Verification items for this drawing (mm, ordinates from the low corner). A direction names the side the tool comes from. Round coordinates to 2 decimals unless told otherwise and drop trailing zeros. Loops run counter-clockwise (first coordinate to the right, second up) from the corner with the lowest first, then second, coordinate; pieces in that order, holes last. Notation, with made-up numbers: (-10.5, 36.5) -> (23.5, 36.5) arc R14 cw to (23.5, 42.5) -> close; hole circle Ø4 at (35, -28.75). An arc over 180 degrees is marked (long way). One line per question, with ' | ' between items.
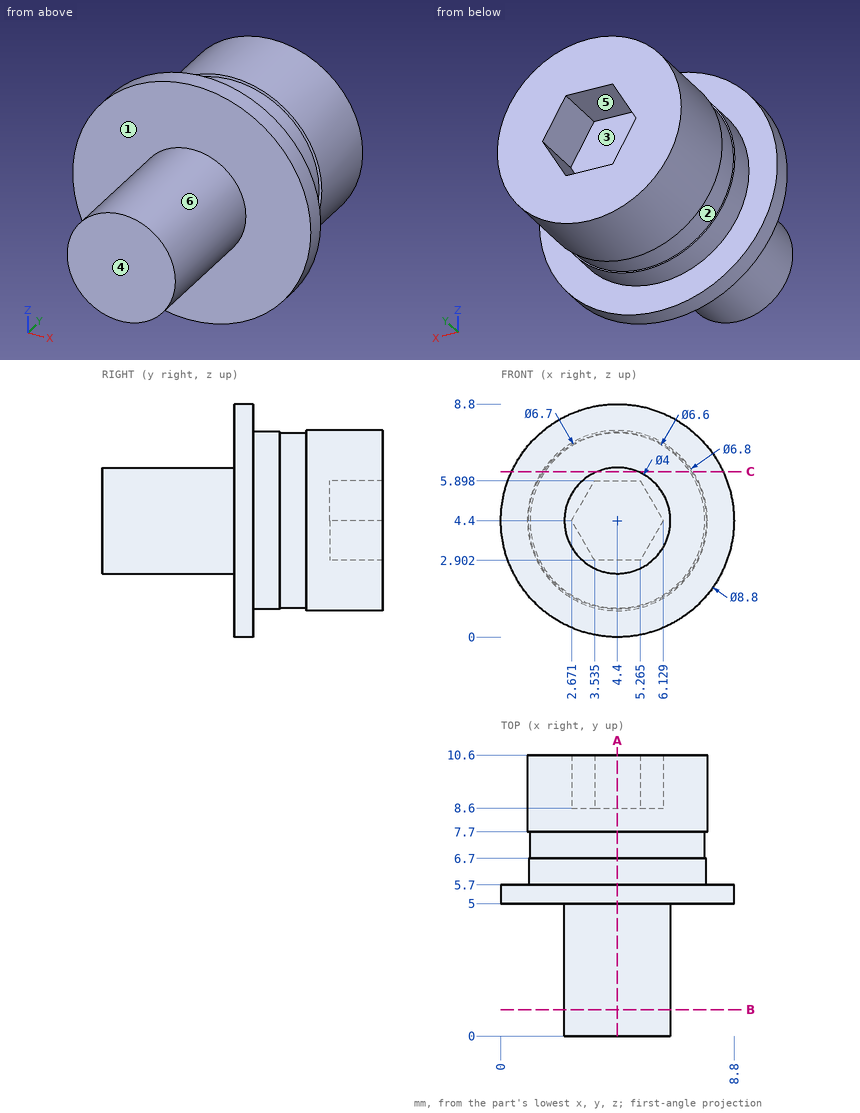
(1) Sectioned sample at A-A, the plane x = 4.4. Record the cut outline in (y, z).
Answer:
outline: (0, 2.4) -> (5, 2.4) -> (5, 0) -> (5.7, 0) -> (5.7, 1.05) -> (6.7, 1.05) -> (6.7, 1.1) -> (7.7, 1.1) -> (7.7, 1) -> (10.6, 1) -> (10.6, 2.9) -> (8.6, 2.9) -> (8.6, 5.9) -> (10.6, 5.9) -> (10.6, 7.8) -> (7.7, 7.8) -> (7.7, 7.7) -> (6.7, 7.7) -> (6.7, 7.75) -> (5.7, 7.75) -> (5.7, 8.8) -> (5, 8.8) -> (5, 6.4) -> (0, 6.4) -> close
(2) Scan lines: probe 1 along Y at (x, z) = (4.75, 4.25); probe 2 along Y at (x, z) = (4.5, 1.25); probe 3 along X at (y, z) = (5.5, 8). Record each from-to range of solid material in increasing order.
Answer:
probe 1: y = 0 to 8.6 | probe 2: y = 5 to 10.6 | probe 3: x = 1.87 to 6.93
(3) Go/stop test with flat-tipped pins: pin 1 (1.4 mm diameter, centred on x = 4, y = 9.5, fed in from +Z); pin 2 (1.9 mm diameter, centred on x = 4, y = 9, fed in from -Z); pin 3 (1.5 mm diameter, centred on x = 4, y = 6, fed in from +Z). Record where each tip stops, or that it passes through.
Answer:
pin 1: stops at z = 7.8 | pin 2: stops at z = 1 | pin 3: stops at z = 8.8
(4) Set-up check for the marked faces 1, 2 and 3: record each of +Z, -Z, +X, -X, +Y, -Y from which the full face is reachable in a straight line by a thin tool's end or side.
Answer:
face 1: -Y | face 2: none | face 3: +Y
(5) Mould release check, pull along Z, two halves, no side actions. Record for the marked faces 4, 5 and 6: +Z half, -Z half, draft (parallel to the pull), parting line (faces both ways), or undercut.
Answer:
face 4: draft | face 5: undercut | face 6: parting line
(6) Sectioned sample at B-B, the plane y = 1. Record the cut outline in (x, z), and give its area (3 significant figures).
Answer:
outline: circle Ø4 at (4.4, 4.4) | area: 12.6 mm2
(7) Sectioned sample at C-C, the plane z = 6.25. Record the cut outline in (x, y), and give its area (3 significant figures).
Answer:
outline: (0.41, 5) -> (3.64, 5) -> (3.64, 0) -> (5.16, 0) -> (5.16, 5) -> (8.39, 5) -> (8.39, 5.7) -> (7.19, 5.7) -> (7.19, 6.7) -> (7.13, 6.7) -> (7.13, 7.7) -> (7.25, 7.7) -> (7.25, 10.6) -> (1.55, 10.6) -> (1.55, 7.7) -> (1.67, 7.7) -> (1.67, 6.7) -> (1.61, 6.7) -> (1.61, 5.7) -> (0.41, 5.7) -> close | area: 40.8 mm2
